```python
from build123d import *

# Parameters (mm, degrees)
SKETCH2_R           = 4.5
FILLET2_R           = 4
SKETCH4_R           = 2
BOSS_EXTRUDE1_DEPTH = 6


with BuildPart() as part:
    # Sweep3: sweep along a path in Sketch3
    with BuildLine(Plane(origin=(0, 0, 0), x_dir=(0, 0, -1), z_dir=(1, 0, 0))) as sweep3_path:
        Line((0, 0), (-25, 0))
        ThreePointArc((-25, 0), (-29.217732486, 1.747041998), (-30.964774484, 5.964774484))
        Line((-30.964774484, 5.964774484), (-30.964774484, 45.964774484))
    # Sketch2 → Sweep3 (sweep)
    with BuildSketch(Plane.XY):
        Circle(SKETCH2_R)
    sweep(path=sweep3_path.line)

    # Fillet2
    fillet2_edges = [part.edges().sort_by_distance(p)[0] for p in [
        (-4.5, 45.964774484, 30.964774484),
    ]]
    fillet(fillet2_edges, radius=FILLET2_R)

    # Sketch4 → Boss-Extrude1 (add)
    with BuildSketch(Plane(origin=(0, 0, 0), x_dir=(0, 0, -1), z_dir=(1, 0, 0))):
        with Locations((-31, 35)):
            Circle(SKETCH4_R)
    extrude(amount=BOSS_EXTRUDE1_DEPTH)


solid = part.part
```
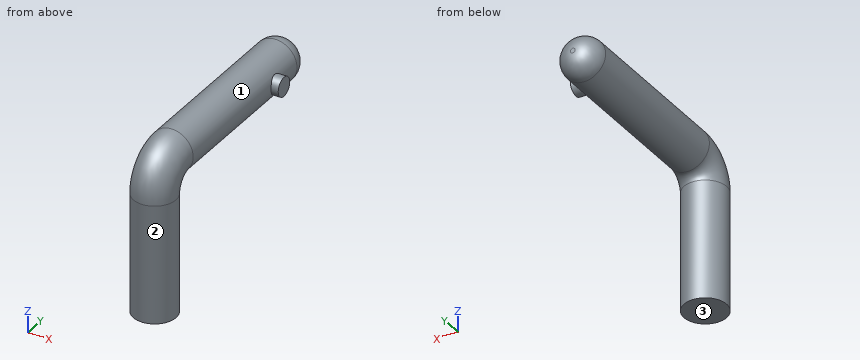
Geometry check sheet. Reference: the model listing, model coordinates, mm. Face numbers are marked on the shaded views. A direction names the side the tool comes from. Round coordinates to 2 decimals unless told otherwise and drop trailing zeros. Loops run counter-clockwise (first coordinate to the right, second up) from the corner with the lowest first, then second, coordinate; pieces in that order, holes last. Notation, with made-up numbers: (-15.5, 72.25) - (-6.5, 72.25) arc R20 cw to (-6.5, 109.25) - close; hole circle Ø4 at (-30.75, 61.25). An arc over 180 degrees is marked (long way). Use a Markdown table: item, result.
Q1. Go/stop test with flat-tipped pins: P1, Ø8, axis at y = 30.5, z = 23.5, coming from the -X side; P2, Ø10, axis at y = 27, z = 28.5, coming from the -X side; P3, Ø4, axis at x = -1.5, y = 28, coming from the -Z side. Record where each tip stops, or that it passes through.
Solutions:
| item | result |
|---|---|
| P1 | stops at x = -2.87 |
| P2 | stops at x = -4.5 |
| P3 | stops at z = 26.46 |
Q2. Material ranges on line 1 (Y direction, x = 0.25, z = 14.5); line 2 (X direction, y = 41, z = 33); line 3 (Y direction, x = -3, z = 3.5), recorded low to high.
Solutions:
| item | result |
|---|---|
| line 1 | y = -4.49 to 4.49 |
| line 2 | x = -4.01 to 4.01 |
| line 3 | y = -3.35 to 3.35 |
Q3. Access from +Z, -Z, +X, -X, +Y, -Y to the whole of each face (thin tool, end or side, straight path). Record for the marked faces 1, 2 and 3.
Solutions:
| item | result |
|---|---|
| face 1 | none |
| face 2 | -Z |
| face 3 | -Z, +X, -X, +Y, -Y |
Q4. Cross-section at C-C on y = 34. Record the cut outline in (x, z), plus the area to 3 significant figures.
Solutions:
| item | result |
|---|---|
| outline | (4.14, 32.73) arc R4.5 ccw (long way) to (4.17, 29.27) - (6, 29.27) - (6, 32.73) - close |
| area | 69.2 mm2 |
Q5. Cross-section at A-A on z = 22.5. Record the cut outline in (x, y).
Solutions:
| item | result |
|---|---|
| outline | circle Ø9 at (0, 0) |
Q6. Cross-section at B-B on y = 15.5. Record the cut outline in (x, z).
Solutions:
| item | result |
|---|---|
| outline | circle Ø9 at (0, 30.96) |
